The figure shows three views and two pictorial views of one solid part (mm, origin at its lowest corner). Answer the questions. Give positions to 0.01 mm unless a question says otherwise; leave off trailing zeros. Loops run counter-clockwise (first coordinate to the right, second up) from the corner with the lowest first, then second, coordinate; pieces in that order, holes last. Notation, with made-up numbers: (56.5, 38) - (105.5, 38) arc R34 ccw to (105.5, 71) - close; hole circle Ø11 at (16.25, -11.75). An arc over 180 degrees is marked (long way). Use CSV: the item, a comma, the result in double quotes.
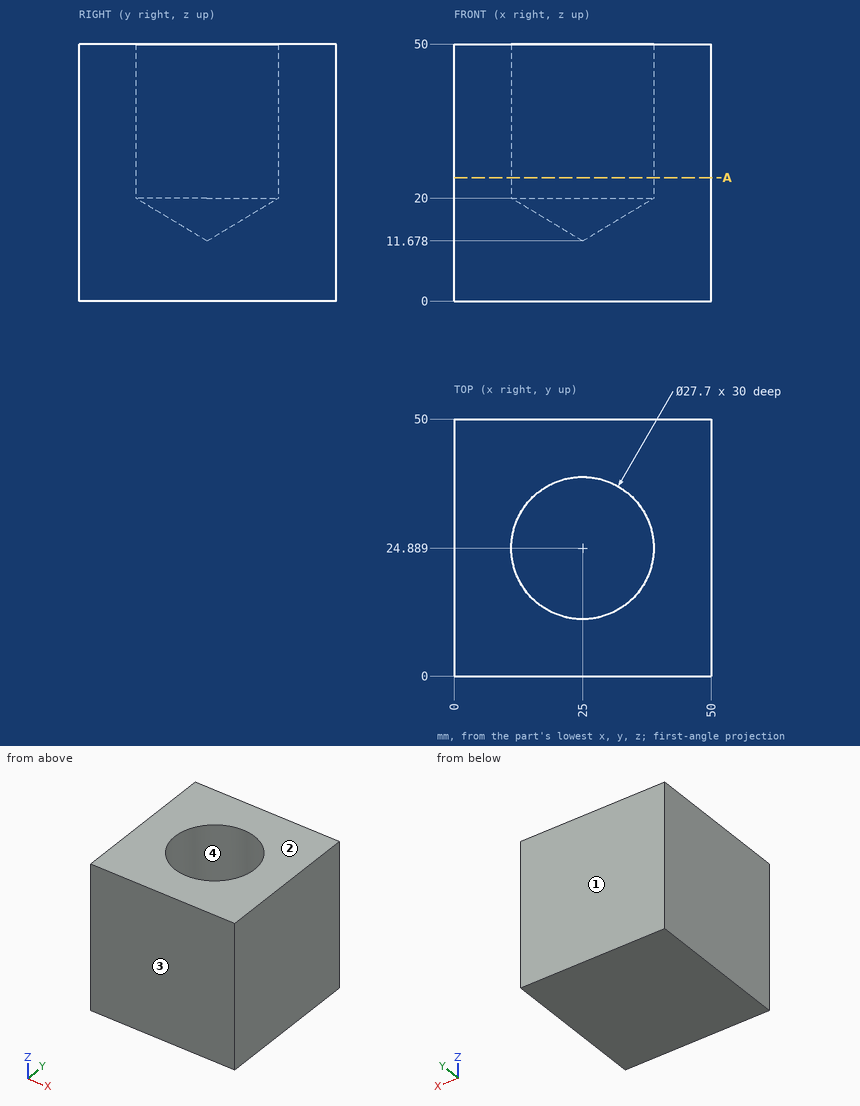
Item 1: Given P1, Ø16.5, axis at x = 25, y = 24.89, coming from the +Z side (1 decimal), flat-ended and moving along its own axis, determine where the tip first touches the part or whether it passes through.
Determined:
P1,"stops at z = 16.6"
Item 2: Find the intervals of material crossed by line 1 (Y direction, x = 25, z = 22); line 2 (X direction, y = 29, z = 41.5) (1 decimal); line 3 (Y direction, x = 37, z = 34) (1 decimal), in increasing order.
Determined:
line 1,"y = 0 to 11.04, 38.74 to 50"
line 2,"x = 0 to 11.8, 38.2 to 50"
line 3,"y = 0 to 18, 31.8 to 50"
Item 3: A cutting plane is placed at A-A on z = 24. Determine the outline of the cut face in (x, y).
Determined:
outline,"(0, 0) - (50, 0) - (50, 50) - (0, 50) - close; hole circle Ø27.7 at (25, 24.89)"
Item 4: The mould has two halves that part along Y. Classify the marked faces 1, 2, 3 and 4: pulls with the +Y half, pulls with the -Y half, needs draft (parallel to the pull), parting line crosses it, or undercut.
Determined:
face 1,"pulls with the +Y half"
face 2,"needs draft"
face 3,"pulls with the -Y half"
face 4,"undercut"
